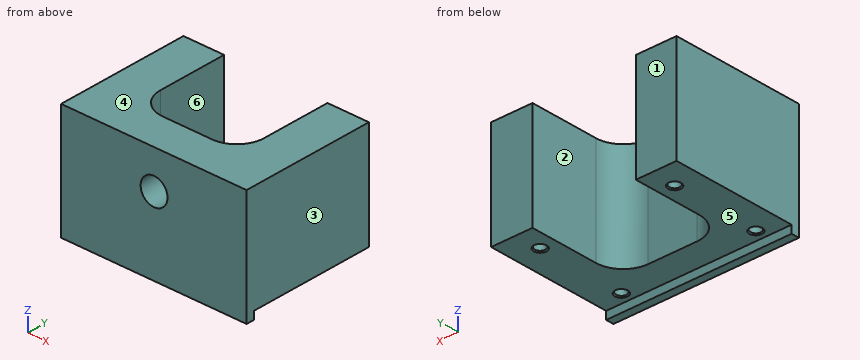
```python
from build123d import *

# Parameters (mm, degrees)
BOSS_EXTRUDE1_DEPTH             = 45.11
CUT_EXTRUDE2_DEPTH              = 100
SKETCH3_R                       = 5.29
CUT_EXTRUDE3_DEPTH              = 100
M5X0_8_TAPPED_HOLE1_D           = 4.2
M5X0_8_TAPPED_HOLE1_DEPTH       = 27.86
M5X0_8_TAPPED_HOLE1_CSINK_D     = 5.05
M5X0_8_TAPPED_HOLE1_CSINK_ANGLE = 90
M5X0_8_TAPPED_HOLE1_TIP         = 1.2618073


with BuildPart() as part:
    # Sketch1 → Boss-Extrude1 (new body)
    with BuildSketch(Plane.XY):
        with BuildLine():
            Line((0, 0), (72.96, 0))
            Line((72.96, 0), (72.96, 52.57))
            Line((72.96, 52.57), (56.67, 52.57))
            Line((56.67, 52.57), (56.67, 25.31))
            ThreePointArc((56.67, 25.31), (53.533113627, 17.736886373), (45.96, 14.6))
            Line((45.96, 14.6), (26.7, 14.6))
            ThreePointArc((26.7, 14.6), (19.126886373, 17.736886373), (15.99, 25.31))
            Line((15.99, 25.31), (15.99, 52.58))
            Line((15.99, 52.58), (0, 52.58))
            Line((0, 52.58), (0, 0))
        make_face()
    extrude(amount=-BOSS_EXTRUDE1_DEPTH)

    # Sketch2 → Cut-Extrude2 (cut)
    with BuildSketch(Plane(origin=(72.96, 0, 0), x_dir=(0, 0, -1), z_dir=(1, 0, 0))):
        Polygon((45.11, 52.57), (45.11, 3.13), (42.05, 3.13), (42.05, 52.57), (42.05, 55.677110027), (45.11, 55.677110027), align=None)
    extrude(amount=-CUT_EXTRUDE2_DEPTH, mode=Mode.SUBTRACT)

    # Sketch3 → Cut-Extrude3 (cut)
    with BuildSketch(Plane.XZ):
        with Locations(Location((36.57, -14.97, 0), (0, 0, 270))):
            Circle(SKETCH3_R)
    extrude(amount=-CUT_EXTRUDE3_DEPTH, mode=Mode.SUBTRACT)

    # M5x0.8 Tapped Hole1
    with Locations(Plane(origin=(0, 0, -42.05), x_dir=(-1, 0, 0), z_dir=(0, 0, -1))):
        with Locations((-62.965, 42.405), (-62.965, 7.5), (-10.06, 7.5), (-10.06, 42.405)):
            CounterSinkHole(M5X0_8_TAPPED_HOLE1_D / 2, M5X0_8_TAPPED_HOLE1_CSINK_D / 2, depth=M5X0_8_TAPPED_HOLE1_DEPTH, counter_sink_angle=M5X0_8_TAPPED_HOLE1_CSINK_ANGLE)
            with Locations((0, 0, -(M5X0_8_TAPPED_HOLE1_DEPTH + M5X0_8_TAPPED_HOLE1_TIP / 2))):  # 118° drill point
                Cone(0, M5X0_8_TAPPED_HOLE1_D / 2, M5X0_8_TAPPED_HOLE1_TIP, mode=Mode.SUBTRACT)


solid = part.part
```
Can you work these out from the model? Positions are in its coordinate system, mm. Face numbers are marked on the shaded views. A direction names the side the tool comes from. Round coordinates to 2 decimals unless told otherwise and drop trailing zeros. Order: outer loops, then holes, each group sorted by start corner. A loop starts at its lowest first (then second) coordinate and runs counter-clockwise, first axis right, second up. Notation, with made-up numbers: (15.5, 27) -> (70.5, 27) arc R17 cw to (70.5, 53) -> close; hole circle Ø10 at (-8.75, -16). An arc over 180 degrees is marked (long way). Return JSON: item names as keys, results as strings. Group by question number.
1. If we section it at B-B, the plane y = 46: Write out the boundary of the cut face in (x, z).
2. Will these pins go through, and if not, where does the flat tip stop? pin 1 (9.5 mm diameter, centred on x = 39.5, z = -31.5, fed in from +Y); pin 2 (18 mm diameter, centred on x = 66, z = -25, fed in from +Y); pin 3 (3 mm diameter, centred on x = 19.5, z = -32, fed in from +Y).
3. I need wall thicknesses on line 1 (X direction, y = 7.5, z = -28) (3 decimals); line 2 (X direction, y = 42.5, z = -36.5); line 3 (Y direction, x = 10, z = -33). Which ranges of each line are inside material? Lowest first, please. Write a range as [from, to].
4. We'd pull the mould along X, two halves only. Please class the marked faces 1, 2 and 3: released by +X, released by -X, zero draft, split by the parting line, or undercut.
5. Which directions (+Z, -Z, +X, -X, +Y, -Y) give clear straight access to the entire face, cutting with the end or side of a thin tool? Please do the marked faces 4, 5 and 6.
6. If we section it at D-D, the plane z = -8: Write out the boundary of the cut face in (x, y).
7. If we section it at C-C, the plane z = -15: Write out the boundary of the cut face in (x, y) (3 decimals).
8. If we section it at A-A, the plane x = 36.57: Write out the boundary of the cut face in (y, z), then the cut area to 3 significant figures.
Output values:
{
 "1": {"outline": "(0, -42.05) -> (15.99, -42.05) -> (15.99, 0) -> (0, 0) -> close; (56.67, -42.05) -> (72.96, -42.05) -> (72.96, 0) -> (56.67, 0) -> close"},
 "2": {"pin 1": "y = 14.6", "pin 2": "y = 52.57", "pin 3": "y = 19.06"},
 "3": {"line 1": "[0, 7.96], [12.16, 60.865], [65.065, 72.96]", "line 2": "[0, 7.96], [12.16, 15.99], [56.67, 60.87], [65.06, 72.96]", "line 3": "[0, 5.4], [9.6, 40.31], [44.5, 52.58]"},
 "4": {"face 1": "zero draft", "face 2": "undercut", "face 3": "released by +X"},
 "5": {"face 4": "+Z, +X, -X, +Y, -Y", "face 5": "-Z, +X, -X, +Y", "face 6": "+Z, -Z, +Y"},
 "6": {"outline": "(0, 0) -> (72.96, 0) -> (72.96, 52.57) -> (56.67, 52.57) -> (56.67, 25.31) arc R10.71 cw to (45.96, 14.6) -> (26.7, 14.6) arc R10.71 cw to (15.99, 25.31) -> (15.99, 52.58) -> (0, 52.58) -> close"},
 "7": {"outline": "(0, 0) -> (31.28, 0) -> (31.28, 14.6) -> (26.7, 14.6) arc R10.71 cw to (15.99, 25.31) -> (15.99, 52.58) -> (0, 52.58) -> close; (41.86, 0) -> (72.96, 0) -> (72.96, 52.57) -> (56.67, 52.57) -> (56.67, 25.31) arc R10.71 cw to (45.96, 14.6) -> (41.86, 14.6) -> close; hole circle Ø4.2 at (10.06, 7.5); hole circle Ø4.2 at (10.06, 42.405); hole circle Ø4.2 at (62.965, 7.5); hole circle Ø4.2 at (62.965, 42.405)"},
 "8": {"outline": "(0, -45.11) -> (3.13, -45.11) -> (3.13, -42.05) -> (14.6, -42.05) -> (14.6, -20.26) -> (0, -20.26) -> close; (0, -9.68) -> (14.6, -9.68) -> (14.6, 0) -> (0, 0) -> close", "area": "469 mm²"}
}
